Autodesk Inventor part; units mm, degrees
ref_plane "YZ Plane" through (0, 0, 0) normal (1, 0, 0) x (0, 1, 0)
ref_plane "XZ Plane" through (0, 0, 0) normal (0, 1, 0) x (-1, 0, 0)
ref_plane "XY Plane" through (0, 0, 0) normal (0, 0, 1) x (1, 0, 0)
sketch "Sketch1" plane through (0, 0, 0) normal (1, 0, 0) x (0, 1, 0)
  circle A0 centre (0, 0) radius 57.5
  dimension "d0" = 115
extrude "Extrusion1" add sketch "Sketch1" along normal blind 2
sketch "Sketch2" plane through (2, 0, 0) normal (1, 0, 0) x (0, 0, -1)
  circle A0 centre (0, 0) radius 58.5
  dimension "d3" = 117
extrude "Extrusion2" add sketch "Sketch2" along normal blind 1
sketch "Sketch3" plane through (0, 0, 0) normal (-1, 0, 0) x (0, 0, 1)
  circle A0 centre (0, 0) radius 58.5
extrude "Extrusion3" add sketch "Sketch3" along normal blind 1
sketch "Sketch4" plane through (-1, 0, 0) normal (-1, 0, 0) x (0, 0, 1)
  circle A0 centre (0, 0) radius 54
  dimension "d8" = 108
extrude "Extrusion4" cut sketch "Sketch4" against normal blind 5
sketch "Sketch5" plane through (-1, 0, 0) normal (-1, 0, 0) x (0, 0, 1)
  circle A0 centre (0, 0) radius 1.5
  circle A1 centre (0, 0) radius 3.5
  dimension "d11" = 3
  dimension "d12" = 7
extrude "Extrusion5" add sketch "Sketch5" against normal blind 5
sketch "Sketch6" plane through (-1, 0, 0) normal (-1, 0, 0) x (0, 0, 1)
  line L0 (2.7345, 0) -> (2.7345, 2) construction
  line L1 (2.7345, 2) -> (2.7345, -2) construction
  line L2 (2.7345, -2) -> (54.8201, -2)
  line L3 (54.8201, -2) -> (54.8201, 2)
  line L4 (54.8201, 2) -> (2.7345, 2)
  line L5 (2.7345, 2) -> (2.7345, -2)
  point P0 (0, 0)
  dimension "d15" = 2
  dimension "d16" = 4
extrude "Extrusion6" add sketch "Sketch6" against normal blind 4
pattern_circular "Circular Pattern1" count 4 over 360 about axis through (-1, 0, 0) along (1, 0, 0) of "Extrusion6"
sketch "Sketch7" plane through (-1, 0, 0) normal (-1, 0, 0) x (0, 0, 1)
  circle A0 centre (0, 0) radius 1.5
  circle A1 centre (0, 0) radius 4
  dimension "d22" = 8
extrude "Extrusion7" add sketch "Sketch7" against normal blind 15
properties part number "mtv_pushingWheel_1-13"
The model under review builds one solid part; all positions refer to its coordinate system, in mm. A direction names the side the tool comes from. Give positions to 0.01 mm unless a question says otherwise; leave off trailing zeros. Order: outer loops, then holes, each group sorted by start corner. A loop starts at its lowest first (then second) coordinate and runs counter-clockwise, first axis right, second up. Notation, with made-up numbers: M 30,2.25 L 81,2.25 A10 ccw 81,9.25 Z; hole C -10,-14 d8. An arc over 180 degrees is marked long. Use one line per item in the form item = value. Start each with the question number.
Item 1: We need section C-C on y = 22.5. Give the boundary of the cut face in (x, z), plus the area to 3 significant figures.
Item 2: To check wall thickness, follow line 1 along Z through (x, y) = (-0.25, -10); line 2 along Y through (x, z) = (4, 0); line 3 along Z through (x, y) = (0.25, -23.5). State the ranges of each line that lie inside material, in increasing order. Write a range as from..to.
Item 3: For faces 1 (the flat face through (-1, 0, 4)), 2 (the cylindrical face through (8.06, 2.7, -2.95)), 3 (the cylindrical face through (0.986, -12.465, 56.133)), 4 (the flat face through (1, -29, 2)), list the 3-axis set-ups (+Z, -Z, +X, -X, +Y, -Y) from which the entire face can be reached by the end or side of a thin tool; tool diameter is ignored.
Item 4: We need section D-D on z = 51.5. Give the boundary of the cut face in (x, y), plus the area to 3 significant figures.
Item 5: Insertion check: pin 1 Ø3 at (x, z) = (0.5, -31) entering from +Y; pin 2 Ø1.2 at (x, z) = (1, -37) entering from -Y; pin 3 Ø1.2 at (x, y) = (2, -29) entering from +Z. Each pin has a flat end and moves straight along its axis. Give the tip position at first contact, or say it passes through.
Item 6: The part is to be moulded in two halves that separate along Z. For faces 5 (the flat face through (14, 0, 2)), 6 (the flat face through (1, 29, -2)), 7 (the cylindrical face through (-0.49, 57.11, -12.68)), say which applies: pulls with the +Z half, pulls with the -Z half, needs draft (parallel to the pull), parting line crosses it, or undercut.
Item 7: We need section A-A on z = 0. Give the boundary of the cut face in (x, y), plus the area to 3 significant figures.
Completed:
q1.outline = M -1,-54 L 0,-54 L 0,-52.92 L 2,-52.92 L 2,-54 L 3,-54 L 3,-49.09 L -1,-49.09 Z; M -1,-2 L 3,-2 L 3,2 L -1,2 Z; M -1,49.09 L 3,49.09 L 3,54 L 2,54 L 2,52.92 L 0,52.92 L 0,54 L -1,54 Z
q1.area = 50.9 mm²
q2.line_1 = -57.64..-53.07, -2..2, 53.07..57.64
q2.line_2 = -4..-1.5, 1.5..4
q2.line_3 = -52.48..-48.62, -2..2, 48.62..52.48
q3.face_1 = +Z, -Z, -X, +Y, -Y
q3.face_2 = +X
q3.face_3 = none
q3.face_4 = +X, -X
q4.outline = M -1,-27.75 L 0,-27.75 L 0,-25.57 L 2,-25.57 L 2,-27.75 L 3,-27.75 L 3,-16.24 L -1,-16.24 Z; M -1,-2 L 3,-2 L 3,2 L -1,2 Z; M -1,16.24 L 3,16.24 L 3,27.75 L 2,27.75 L 2,25.57 L 0,25.57 L 0,27.75 L -1,27.75 Z
q4.area = 99.4 mm²
q5.pin_1 = 50.47
q5.pin_2 = -44.51
q5.pin_3 = 51.14
q6.face_5 = needs draft
q6.face_6 = undercut
q6.face_7 = parting line crosses it
q7.outline = M -1,-58.5 L 0,-58.5 L 0,-57.5 L 2,-57.5 L 2,-58.5 L 3,-58.5 L 3,-4 L 14,-4 L 14,-1.5 L -1,-1.5 Z; M -1,1.5 L 14,1.5 L 14,4 L 3,4 L 3,58.5 L 2,58.5 L 2,57.5 L 0,57.5 L 0,58.5 L -1,58.5 Z
q7.area = 507 mm²
